Source: CAD feature listing. Evaluate the final solid. Frame: model axes, mm. Round coordinates to 2 decimals unless told otherwise and drop trailing zeros. Order: outer loops, then holes, each group sorted by start corner. A loop starts at its lowest first (then second) coordinate and runs counter-clockwise, first axis right, second up. Notation, with made-up numbers: (63.25, 44.25) -> (111.25, 44.25) arc R32 ccw to (111.25, 75.25) -> close; hole circle Ø11 at (-17.5, 56.25). An arc over 180 degrees is marked (long way). Write item = value, one per line. Start each with the question number.
(1) Cut plane A-A on z = 0. Return the cut outline in (x, y), then the cut area to 3 significant figures.
(2) Ray query, line 1 (Y direction, x = -2.5, z = 0.15); line 2 (Z direction, x = 10.5, y = -181); line 3 (X direction, y = -141.5, z = -0.75). Return the intervals inside material, ascending.
(3) Contact query for flat-ended pins moving along their axis: pin 1 Ø2 at (y, z) = (-128, -1) entering from -X; pin 2 Ø3 at (x, y) = (-1.5, -90) entering from +Z; pin 3 Ø5 at (x, y) = (4.5, -108.5) entering from -Z. Output: stop coordinate, or through.
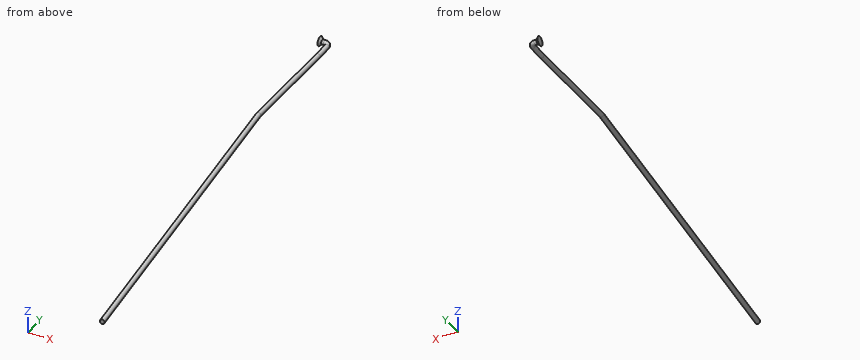
from build123d import *

# Parameters (mm, degrees)
ESQUISSE2_R = 1


with BuildPart() as part:
    # Balayage1: sweep along a path in Esquisse1
    with BuildLine(Plane.XY) as balayage1_path:
        Line((12.194958481, -203.034093166), (-1.177962674, -53.984579624))
        Line((-1.177962674, -53.984579624), (0, -9))
        Line((0, -9), (0, -2))
        ThreePointArc((0, -2), (-0.585786438, -0.585786438), (-2, 0))
        Line((-2, 0), (-4, 0))
    # Esquisse2 → Balayage1 (sweep)
    with BuildSketch(Plane(origin=(-4, 0, 0), x_dir=(0, 0, -1), z_dir=(1, 0, 0))):
        Circle(ESQUISSE2_R)
    sweep(path=balayage1_path.line, transition=Transition.RIGHT)

    # Esquisse3 → Révolution1 (revolve)
    with BuildSketch(Plane.XY):
        Polygon((-4, 1), (-4, 2), (-3, 1), align=None)
    revolve(axis=Axis((0, 0, 0), (-1, 0, 0)))


solid = part.part
Evaluation:
q1.outline = (-4, -2) -> (-3, -1) -> (-2, -1) arc R1 cw to (-1, -2) -> (-1, -8.99) -> (-2.18, -54.02) -> (11.2, -203.12) -> (13.19, -202.94) -> (-0.18, -53.95) -> (1, -9.01) -> (1, -2) arc R3 ccw to (-2, 1) -> (-3, 1) -> (-4, 2) -> close
q1.area = 415 mm^2
q2.line_1 = -0.99 to 0.99
q2.line_2 = -0.96 to 0.96
q2.line_3 = 6.01 to 7.34
q3.pin_1 = 4.42
q3.pin_2 = through
q3.pin_3 = -1
